The model under review builds one solid part; all positions refer to its coordinate system, in mm. Face numbers are marked on the shaded views. Give positions to 0.01 mm unless a question says otherwise; leave off trailing zeros. Order: outer loops, then holes, each group sorted by start corner. A loop starts at its lowest first (then second) coordinate and runs counter-clockwise, first axis right, second up. Notation, with made-up numbers: (54, -7) - (110, -7) arc R33 cw to (110, 26) - close; hole circle Ø9 at (76.25, 18). An arc over 180 degrees is marked (long way). Use CSV: the item, a comma, the result in double quotes.
Autodesk Inventor part; units mm, degrees
ref_plane "YZ Plane" through (0, 0, 0) normal (1, 0, 0) x (0, 1, 0)
ref_plane "XZ Plane" through (0, 0, 0) normal (0, 1, 0) x (-1, 0, 0)
ref_plane "XY Plane" through (0, 0, 0) normal (0, 0, 1) x (1, 0, 0)
sketch "Sketch1" plane through (0, 0, 0) normal (1, 0, 0) x (0, 1, 0)
  line L0 (-19.5584, -4) -> (19.5584, -4)
  line L1 (19.5584, -4) -> (19.5584, 4)
  line L2 (19.5584, 4) -> (-19.5584, 4)
  line L3 (-19.5584, 4) -> (-19.5584, -4)
  line L4 (-19.5584, -4) -> (19.5584, 4) construction
  line L5 (19.5584, -4) -> (-19.5584, 4) construction
  point P0 (0, 0)
  dimension "d0" = 8
extrude "Extrusion1" add sketch "Sketch1" along normal blind 7
sketch "Sketch2" plane through (7, 0, 0) normal (1, 0, 0) x (0, 0, -1)
  arc A0 (4, 15.5584) -> (-4, 15.5584) centre (0, 15.5584) ccw
  point P0 (0, 0)
fillet "Fillet2" radius 4 2 edges at (3.5, 19.5584, -4) (3.5, 19.5584, 4)
hole "Hole1" at (7, 15.5584, 0) direction (-1, 0, 0) diameter 3 end through all
sketch "Sketch3" plane through (0, -19.5584, 4) normal (0, 0, 1) x (1, 0, 0)
  line L0 (0, 0) -> (7, 0)
  point P0 (0, 19.5584)
  point P1 (3.5348, 4)
  dimension "d12" = 4
hole "Hole2" at (3.5348, -15.5584, 4) direction (0, 0, -1) diameter 3 end through all
properties part number "Puller"
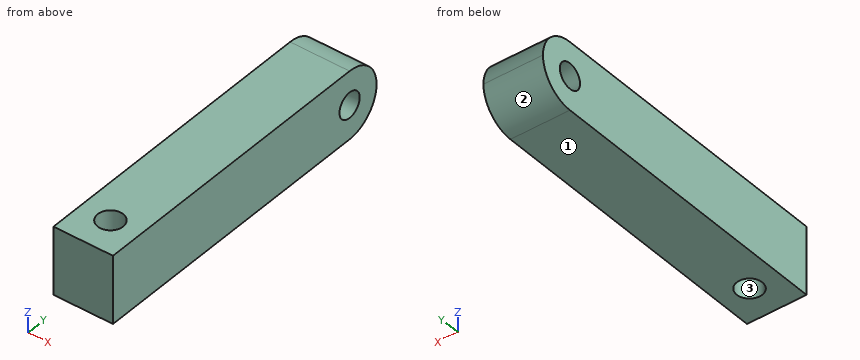
Item 1: Take a section at A-A, the plane z = 1. Give the boundary of the cut face in (x, y), and give its area (3 significant figures).
Results list:
outline,"(0, -19.56) - (7, -19.56) - (7, 14.44) - (0, 14.44) - close; (0, 16.68) - (7, 16.68) - (7, 19.43) - (0, 19.43) - close; hole circle Ø3 at (3.53, -15.56)"
area,"250 mm2"
Item 2: Wall thickness on L1, parallel to Y at x = 2.5, z = 0; L2, parallel to Y at x = 4.25, z = 0.25; L3, parallel to Y at x = 4, z = 2: over which ranges is each line inside the solid? List them lowest first.
Results list:
L1,"y = -19.56 to -16.64, -14.47 to 14.06, 17.06 to 19.56"
L2,"y = -19.56 to -16.88, -14.24 to 14.08, 17.04 to 19.55"
L3,"y = -19.56 to -16.98, -14.13 to 19.02"
Item 3: Mouldability with a two-part tool opening along Y and no side actions: class the marked faces 1, 2 and 3 as pulls with the +Y half, pulls with the -Y half, needs draft (parallel to the pull), parting line crosses it, or undercut.
Results list:
face 1,"needs draft"
face 2,"pulls with the +Y half"
face 3,"undercut"
Item 4: Clearance check with flat-ended pins moving along their axes: pin 1 (2.5 mm diameter, centred on x = 3.53, y = -15.56, fed in from -Z); pin 2 (3 mm diameter, centred on x = 1, z = 2.5, fed in from +Y). State where each tip first meets the part, or that it passes through.
Results list:
pin 1,"passes through"
pin 2,"stops at y = 19.43"
Item 5: Take a section at B-B, the plane z = -3. Give the boundary of the cut face in (x, y), and give its area (3 significant figures).
Results list:
outline,"(0, -19.56) - (7, -19.56) - (7, 18.2) - (0, 18.2) - close; hole circle Ø3 at (3.53, -15.56)"
area,"257 mm2"
Item 6: Take a section at C-C, the plane z = 3.5. Give the boundary of the cut face in (x, y).
Results list:
outline,"(0, -19.56) - (7, -19.56) - (7, 17.5) - (0, 17.5) - close; hole circle Ø3 at (3.53, -15.56)"
